Design review of the part built by this model. Coordinates are the model's own, in mm. Face numbers are marked on the shaded views. A direction names the side the tool comes from. Give positions to 0.01 mm unless a question says otherwise; leave off trailing zeros. Order: outer loops, then holes, each group sorted by start corner. A loop starts at its lowest first (then second) coordinate and runs counter-clockwise, first axis right, second up.
```python
from build123d import *

# Parameters (mm, degrees)
SKETCH_1_W          = 20
SKETCH_1_H          = 20
EXTRUDE_1_DEPTH     = 4
SKETCH_2_W          = 12.9
SKETCH_2_H          = 20
EXTRUDE_2_DEPTH     = 3.8
SKETCH_3_R          = 1.6
CUT_EXTRUDE_1_DEPTH = 30.340074983
SKETCH_4_W          = 5.8
SKETCH_4_H          = 20
SKETCH_4_R          = 1.6
EXTRUDE_3_DEPTH     = 1.5
SKETCH_5_R          = 3
CUT_EXTRUDE_3_DEPTH = 2.4
CHAMFER_3_SIZE      = 1.5
CHAMFER_1_SIZE      = 6.6
CHAMFER_2_SIZE      = 1
CHAMFER_4_SIZE      = 0.4
CHAMFER_5_SIZE      = 0.9


with BuildPart() as part:
    # 草图1 → 凸台-拉伸1 (new body)
    with BuildSketch(Plane(origin=(0, 0, 0), x_dir=(1, 0, 0), z_dir=(0, 1, 0))):
        with Locations((10, 10)):
            Rectangle(SKETCH_1_W, SKETCH_1_H)
    extrude(amount=EXTRUDE_1_DEPTH)

    # 草图2 → 凸台-拉伸2 (add)
    with BuildSketch(Plane(origin=(0, 4, 0), x_dir=(1, 0, 0), z_dir=(0, 1, 0))):
        with Locations((6.45, 10)):
            Rectangle(SKETCH_2_W, SKETCH_2_H)
    extrude(amount=EXTRUDE_2_DEPTH)

    # 草图3 → 切除-拉伸1 (cut, through all)
    with BuildSketch(Plane(origin=(0, 0, 0), x_dir=(-1, 0, 0), z_dir=(0, -1, 0))):
        with Locations(Location((-10, 5, 0), (0, 0, 90))):
            Circle(SKETCH_3_R)
        with Locations(Location((-10, 15, 0), (0, 0, 90))):
            Circle(SKETCH_3_R)
    extrude(amount=-CUT_EXTRUDE_1_DEPTH, mode=Mode.SUBTRACT)

    # 草图4 → 凸台-拉伸3 (add)
    with BuildSketch(Plane(origin=(0, 7.8, 0), x_dir=(1, 0, 0), z_dir=(0, 1, 0))):
        with Locations((10, 10)):
            Rectangle(SKETCH_4_W, SKETCH_4_H)
        with Locations(Location((10, 15, 0), (0, 0, 90))):
            Circle(SKETCH_4_R, mode=Mode.SUBTRACT)
        with Locations(Location((10, 5, 0), (0, 0, 90))):
            Circle(SKETCH_4_R, mode=Mode.SUBTRACT)
    extrude(amount=EXTRUDE_3_DEPTH)

    # 草图5 → 切除-拉伸3 (cut)
    with BuildSketch(Plane(origin=(0, 0, 0), x_dir=(-1, 0, 0), z_dir=(0, -1, 0))):
        with Locations(Location((-10, 5, 0), (0, 0, 90))):
            Circle(SKETCH_5_R)
        with Locations(Location((-10, 15, 0), (0, 0, 90))):
            Circle(SKETCH_5_R)
    extrude(amount=-CUT_EXTRUDE_3_DEPTH, mode=Mode.SUBTRACT)

    # 倒角3
    # the kernel refuses this chamfer: 1.5 mm, written as the material it takes off along each edge
    with BuildSketch(Plane(origin=(10, 2.4, -15), x_dir=(0, 0, -1), z_dir=(-1, 0, 0))) as chamfer_3_piece_1_section:
        Polygon((1.6 + CHAMFER_3_SIZE, 0), (1.6, -CHAMFER_3_SIZE), (1.6, 0), align=None)
    chamfer_3_piece_1 = revolve(axis=Axis((10, 2.4, -15), (0, -1, 0)), mode=Mode.PRIVATE)
    chamfer_3_piece_1 = chamfer_3_piece_1 & Plane(origin=(10, 3.20338318, -15), x_dir=(0, 0, -1), z_dir=(0, -1, 0)) * Cylinder(3, 13, mode=Mode.PRIVATE)
    add(chamfer_3_piece_1, mode=Mode.SUBTRACT)
    with BuildSketch(Plane(origin=(10, 2.4, -5), x_dir=(0, 0, -1), z_dir=(-1, 0, 0))) as chamfer_3_piece_2_section:
        Polygon((1.6 + CHAMFER_3_SIZE, 0), (1.6, -CHAMFER_3_SIZE), (1.6, 0), align=None)
    chamfer_3_piece_2 = revolve(axis=Axis((10, 2.4, -5), (0, -1, 0)), mode=Mode.PRIVATE)
    chamfer_3_piece_2 = chamfer_3_piece_2 & Plane(origin=(10, 3.20338318, -5), x_dir=(0, 0, -1), z_dir=(0, -1, 0)) * Cylinder(3, 13, mode=Mode.PRIVATE)
    add(chamfer_3_piece_2, mode=Mode.SUBTRACT)

    # 倒角1
    chamfer_1_edges = [part.edges().sort_by_distance(p)[0] for p in [
        (0, 0, -10),
    ]]
    chamfer(chamfer_1_edges, length=CHAMFER_1_SIZE)

    # 倒角2
    chamfer_2_edges = [part.edges().sort_by_distance(p)[0] for p in [
        (20, 4, -10),
        (16.45, 4, 0),
        (12.9, 6.65, 0),
        (12.9, 6.65, -20),
        (16.45, 4, -20),
        (20, 0, -10),
    ]]
    chamfer(chamfer_2_edges, length=CHAMFER_2_SIZE)

    # 倒角4
    chamfer_4_edges = [part.edges().sort_by_distance(p)[0] for p in [
        (0, 7.8, -10),
    ]]
    chamfer(chamfer_4_edges, length=CHAMFER_4_SIZE)

    # 倒角5
    chamfer_5_edges = [part.edges().sort_by_distance(p)[0] for p in [
        (7.1, 9.3, -10),
        (12.9, 9.3, -10),
    ]]
    chamfer(chamfer_5_edges, length=CHAMFER_5_SIZE)


solid = part.part
```
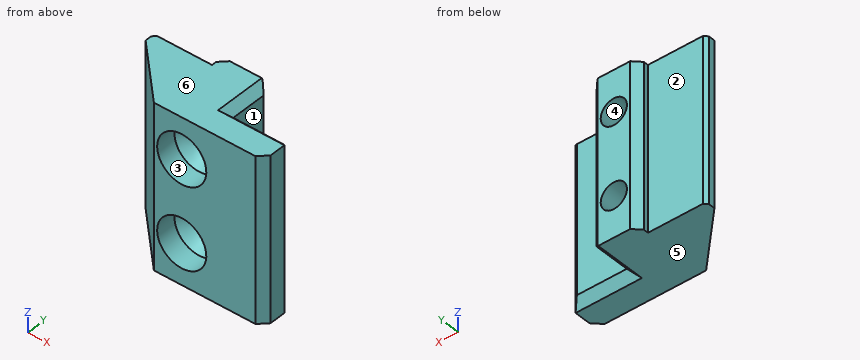
1. Take a section at A-A (x = 10). State the section outline as (y, z) points, then the cut area to 3 significant figures.
Recorded:
outline: (0, -20) - (9.3, -20) - (9.3, -16.6) - (3.9, -16.6) - (2.5, -18) - (0, -18) - close; (0, -12) - (2.5, -12) - (3.9, -13.4) - (9.3, -13.4) - (9.3, -6.6) - (3.9, -6.6) - (2.5, -8) - (0, -8) - close; (0, -2) - (2.5, -2) - (3.9, -3.4) - (9.3, -3.4) - (9.3, 0) - (0, 0) - close
area: 109 mm2
2. Draft analysis for pull direction Z (two halves, no side actions). For the marked faces 4, 5 and 6, state which applies: pulls with the +Z half, pulls with the -Z half, needs draft (parallel to the pull), parting line crosses it, or undercut.
Recorded:
face 4: undercut
face 5: pulls with the -Z half
face 6: pulls with the +Z half
3. For pin 1 (2 mm diameter, centred on x = 5, z = -14, fed in from +Y); pin 2 (5.5 mm diameter, centred on x = 10, z = -5, fed in from -Y); pin 3 (3.5 mm diameter, centred on y = 5.5, z = -7, fed in from +X); pin 4 (1.9 mm diameter, centred on x = 10, z = -5, fed in from -Y), all flat-tipped, find the tip position at first contact; note any pin that passes through.
Recorded:
pin 1: stops at y = 7.8
pin 2: stops at y = 2.75
pin 3: stops at x = 19.25
pin 4: passes through
4. Take a section at B-B (y = 5.5). State the section outline as (x, z) points.
Recorded:
outline: (1.1, -20) - (11.9, -20) - (12.9, -19) - (12.9, -1) - (11.9, 0) - (1.1, 0) - close; hole circle Ø3.2 at (10, -15); hole circle Ø3.2 at (10, -5)
5. For line 1 along Z through (x, y) = (10, 6.2); line 2 along Y through (x, z) = (13.25, -6); line 3 along Y through (x, z) = (6.75, -0.75), list the stretches that pass through material, from the lowest coordinate up.
Recorded:
line 1: z = -20 to -16.6, -13.4 to -6.6, -3.4 to 0
line 2: y = 0 to 4
line 3: y = 0 to 7.8
6. Take a section at C-C (z = -5). State the section outline as (x, y) points, then the cut area to 3 significant figures.
Recorded:
outline: (0, 6.6) - (6.6, 0) - (7, 0) - (7, 2.5) - (8.4, 3.9) - (8.4, 9.3) - (8, 9.3) - (7.1, 8.4) - (7.1, 7.8) - (0.4, 7.8) - (0, 7.4) - close; (11.6, 3.9) - (13, 2.5) - (13, 0) - (19, 0) - (20, 1) - (20, 3) - (19, 4) - (12.9, 4) - (12.9, 8.4) - (12, 9.3) - (11.6, 9.3) - close
area: 75.3 mm2
7. Machinability: for the marked faces 1, 2 and 3, which of the approach directions +Z, -Z, +X, -X, +Y, -Y give a long, thin tool a straight path to every point of the face, cutting with its end or side? Answer none if there is none.
Recorded:
face 1: +Z, -Z, +X, +Y
face 2: +Z, -Z, -X, +Y
face 3: -Y
8. Take a section at D-D (z = -10.75). State the section outline as (x, y) points, then the cut area to 3 significant figures.
Recorded:
outline: (0, 6.6) - (6.6, 0) - (19, 0) - (20, 1) - (20, 3) - (19, 4) - (12.9, 4) - (12.9, 8.4) - (12, 9.3) - (8, 9.3) - (7.1, 8.4) - (7.1, 7.8) - (0.4, 7.8) - (0, 7.4) - close
area: 114 mm2
